Autodesk Inventor part; units mm, degrees
ref_plane "YZ Plane" through (0, 0, 0) normal (1, 0, 0) x (0, 1, 0)
ref_plane "XZ Plane" through (0, 0, 0) normal (0, 1, 0) x (-1, 0, 0)
ref_plane "XY Plane" through (0, 0, 0) normal (0, 0, 1) x (1, 0, 0)
sketch "Boceto1" plane through (0, 0, 0) normal (0, 1, 0) x (-1, 0, 0)
  circle A0 centre (0, 0) radius 6
  dimension "d0" = 0
  dimension "d1" = 0
  dimension "d2" = 12
extrude "Extrusión1" add sketch "Boceto1" along normal blind 15
fillet "Empalme1" radius 5.5 1 edges at (6, 15, 0)
sketch "Boceto2" plane through (0, 0, 0) normal (0, -1, 0) x (1, 0, 0)
  circle A0 centre (0, 0) radius 7.5
  dimension "d6" = 15
extrude "Extrusión2" add sketch "Boceto2" against normal blind 10
fillet "Empalme2" radius 1 1 edges at (-7.5, 10, 0)
sketch "Boceto3" plane through (0, 0, 0) normal (0, -1, 0) x (1, 0, 0)
  circle A0 centre (0, 0) radius 6.5
  circle A1 centre (7.5, 0) radius 2
  circle A2 centre (-7.5, 0) radius 2
  dimension "d10" = 7.5
  dimension "d12" = 4
  dimension "d14" = 7.5
  dimension "d15" = 4
extrude "Extrusión3" add sketch "Boceto3" against normal blind 6.5 contours A0 A1 | A0 A1 | A2 A0 | A0 A2
equation "\"Radio_pliegue\" = Grosor"
equation "\"Anchura_desahogo_plegado\" = Grosor"
equation "\"Profundidad_desahogo_plegado\" = 0.5 * Grosor"
equation "\"Tamaño_destalonado\" = 4 * Grosor"
equation "\"Remanente_mínimo\" = 2 * Grosor"
equation "\"Radiodetransición\" = Radio_pliegue"
equation "\"Tamaño_de_radio_de_Jacobi\" = Radio_pliegue"
equation "\"TamañoSeparación\" = Grosor"
properties part number "Rueda Loca"
Part model, mm, in its own coordinate system. A direction names the side the tool comes from. Round coordinates to 2 decimals unless told otherwise and drop trailing zeros. Write each loop counter-clockwise with the first axis right and the second up, starting at its lowest first coordinate (ties: lowest second). Pieces come first, ordered by that corner, then holes. Notation, with made-up numbers: M 49,-21 L 88,-21 A31 cw 88,16 Z; hole C -18,21.25 d8. An arc over 180 degrees is marked long. Answer as CSV lines item,"result". Start each with the question number.
1) Drop flat-ended pins along their axis: pin 1 (0.7 mm diameter, centred on x = -9, z = 0, fed in from +Y); pin 2 (1.8 mm diameter, centred on x = 8, z = 0.5, fed in from +Y); pin 3 (6 mm diameter, centred on x = -7, y = 4.5, fed in from +Z). Give the stop position or say it passes through.
2) Band-saw the part on A-A (y = 7.5). List the corners of the cut face in (x, z).
3) Band-saw the part on B-B (x = 8). List the corners of the cut face in (y, z).
4) Band-saw the part on C-C (y = 4.5). List the corners of the cut face in (x, z), then the cut area to 3 significant figures.
5) Band-saw the part on D-D (y = 9.25). List the corners of the cut face in (x, z), then the cut area to 3 significant figures.
6) Drill centre lines: L1, parallel to Y at x = 4, z = -5; L2, parallel to Z at x = 0.25, y = 5.75; L3, parallel to X at y = 6, z = -3.75. Where is each one in solid material? Low to high.
7) Which spindle directions (+Z, -Z, +X, -X, +Y, -Y) get a long thin tool onto all of the face, cutting with end or side? Do faces 1 (the face through (6, 10, -2)), 2 (the face through (0, 15, 0)). Say none if no direction does.
Worked out:
1,pin 1,"y = 6.5"
1,pin 2,"y = 9.79"
1,pin 3,"z = 6.34"
2,outline,"C 0,0 d15"
3,outline,"M 0,-1.94 L 6.5,-1.94 L 6.5,1.94 L 0,1.94 Z"
4,outline,"M -7.23,-1.98 A7.5 ccw 7.23,-1.98 A2 ccw long 7.23,1.98 A7.5 ccw -7.23,1.98 A2 ccw long Z"
4,area,"190 mm²"
5,outline,"C 0,0 d14.94"
5,area,"175 mm²"
6,L1,"0 to 10"
6,L2,"-7.5 to 7.5"
6,L3,"-6.5 to 6.5"
7,face 1,"+Y"
7,face 2,"+Z, -Z, +X, -X, +Y"
